from build123d import *

# Parameters (mm, degrees)
BOSS_EXTRUDE1_DEPTH = 16.8656
CHAMFER1_SIZE       = 0.254
SKETCH2_R           = 11.7475
BOSS_EXTRUDE2_DEPTH = 104.521
SKETCH3_R           = 1.5875
CUT_EXTRUDE1_DEPTH  = 16.3576
SKETCH4_R           = 2.286
CUT_EXTRUDE2_DEPTH  = 122.3866


with BuildPart() as part:
    # Sketch1 → Boss-Extrude1 (new body)
    with BuildSketch(Plane(origin=(0, 0, 0), x_dir=(1, 0, 0), z_dir=(0, 1, 0))):
        with BuildLine():
            Line((0, 13.97), (25.4, 13.97))
            ThreePointArc((25.4, 13.97), (39.37, 0), (25.4, -13.97))
            Line((25.4, -13.97), (0, -13.97))
            ThreePointArc((0, -13.97), (-13.97, 0), (0, 13.97))
        make_face()
    extrude(amount=BOSS_EXTRUDE1_DEPTH)

    # Chamfer1
    chamfer1_edges = [part.edges().sort_by_distance(p)[0] for p in [
        (39.37, 16.8656, 0),
        (12.7, 16.8656, -13.97),
        (-13.97, 16.8656, 0),
        (12.7, 16.8656, 13.97),
    ]]
    chamfer(chamfer1_edges, length=CHAMFER1_SIZE)

    # Sketch2 → Boss-Extrude2 (add)
    with BuildSketch(Plane.XZ):
        Circle(SKETCH2_R)
        with Locations((25.4, 0)):
            Circle(SKETCH2_R)
    extrude(amount=BOSS_EXTRUDE2_DEPTH)

    # Sketch3 → Cut-Extrude1 (cut)
    with BuildSketch(Plane(origin=(0, 16.8656, 0), x_dir=(1, 0, 0), z_dir=(0, 1, 0))):
        with Locations((25.4, 6.096)):
            Circle(SKETCH3_R)
        with Locations((31.496, 0)):
            Circle(SKETCH3_R)
        with Locations((25.4, -6.096)):
            Circle(SKETCH3_R)
        with Locations((19.304, 0)):
            Circle(SKETCH3_R)
        with Locations((-6.096, 0)):
            Circle(SKETCH3_R)
        with Locations((6.096, 0)):
            Circle(SKETCH3_R)
        with Locations((0, -6.096)):
            Circle(SKETCH3_R)
        with Locations((0, 6.096)):
            Circle(SKETCH3_R)
    extrude(amount=-CUT_EXTRUDE1_DEPTH, mode=Mode.SUBTRACT)

    # Sketch4 → Cut-Extrude2 (cut, through all)
    with BuildSketch(Plane(origin=(0, 16.8656, 0), x_dir=(1, 0, 0), z_dir=(0, 1, 0))):
        with Locations((12.7, 10.16)):
            Circle(SKETCH4_R)
        with Locations((12.7, -10.16)):
            Circle(SKETCH4_R)
    extrude(amount=-CUT_EXTRUDE2_DEPTH, mode=Mode.SUBTRACT)


solid = part.part
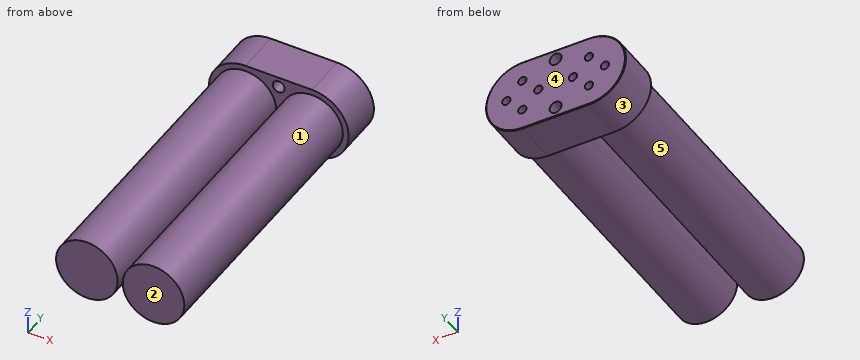
Read the model definition and answer for the solid it produces. Units are mm, in the model's axes. Face numbers are marked on the shaded views. A direction names the side the tool comes from. Give positions to 0.01 mm unless a question says otherwise; leave off trailing zeros. Loops run counter-clockwise (first coordinate to the right, second up) from the corner with the lowest first, then second, coordinate; pieces in that order, holes last. Notation, with made-up numbers: (-29.75, -38.75) -> (-14.75, -38.75) arc R21 cw to (-14.75, -10.75) -> close; hole circle Ø7 at (18, -35). An arc over 180 degrees is marked (long way). Use a Markdown table: item, result.
Q1. A tool of negligible diameter and unlimited length cuts with its end or side. For the marked faces 1 and 2, from which of +Z, -Z, +X, -X, +Y, -Y can it reach the whole face along a straight path? Write none if from no direction.
Solved:
| item | result |
|---|---|
| face 1 | -Y |
| face 2 | +Z, -Z, +X, -X, -Y |
Q2. Section B-B, the plane y = -10.5 is taken. Determine the outline of the cut face in (x, z) (1 decimal), then the cut area to 3 significant figures.
Solved:
| item | result |
|---|---|
| outline | circle Ø23.5 at (0, 0); circle Ø23.5 at (25.4, 0) |
| area | 867 mm^2 |
Q3. Each of these flat-tipped pins is pushed along its axis until it touches: pin 1 (5 mm diameter, centred on y = -81.5, z = 4.5, fed in from +X); pin 2 (12 mm diameter, centred on y = -84, z = 9.5, fed in from +X); pin 3 (3 mm diameter, centred on x = -6.096, z = 0, fed in from +Y). Where does it stop, or does it pass through?
Solved:
| item | result |
|---|---|
| pin 1 | stops at x = 36.98 |
| pin 2 | stops at x = 36.61 |
| pin 3 | stops at y = 0.51 |
Q4. Determine the mould class of the marked faces 3, 4 and 5 for opening direction X: pulls with the +X half, pulls with the -X half, needs draft (parallel to the pull), parting line crosses it, or undercut.
Solved:
| item | result |
|---|---|
| face 3 | pulls with the -X half |
| face 4 | needs draft |
| face 5 | undercut |
Q5. Find the intervals of material crossed by line 1 along Z through (x, y) = (0, 11.5); line 2 along X through (y, z) = (7.25, 0); line 3 along Z through (x, y) = (25, -30.5), in increasing order.
Solved:
| item | result |
|---|---|
| line 1 | z = -13.97 to -7.68, -4.51 to 4.51, 7.68 to 13.97 |
| line 2 | x = -13.97 to -7.68, -4.51 to 4.51, 7.68 to 17.72, 20.89 to 29.91, 33.08 to 39.37 |
| line 3 | z = -11.74 to 11.74 |
